The model under review builds one solid part; all positions refer to its coordinate system, in mm. A direction names the side the tool comes from. Round coordinates to 2 decimals unless told otherwise and drop trailing zeros. Write each loop counter-clockwise with the first axis right and the second up, starting at its lowest first coordinate (ties: lowest second). Pieces come first, ordered by that corner, then holes. Notation, with made-up numbers: (-1.75, 75.25) -> (38.25, 75.25) arc R19 ccw to (38.25, 110.25) -> close; hole circle Ø9 at (-9, 75). An arc over 180 degrees is marked (long way). Answer as a JSON object with one key per item and string values. Group by question number.
1) Insertion check: pin 1 Ø3 at (y, z) = (3, 18) entering from -X; pin 2 Ø3 at (x, y) = (4, 3) entering from +Z; pin 3 Ø3 at (x, y) = (5.5, 5) entering from +Z. Each pin has a flat end and moves straight along its axis. Give the tip position at first contact, or say it passes through.
2) Mouldability with a two-part tool opening along Z and no side actions: class faces 3 (the flat face through (-20, 6.35, -1)), 4 (the cylindrical face through (37.26, 3.13, -12.29)), 5 (the cylindrical face through (-46.492, 3.131, -10.324)) as pulls with the +Z half, pulls with the -Z half, needs draft (parallel to the pull), parting line crosses it, or undercut.
3) Machinability: for faces 1 (the cylindrical face through (12.495, 3.219, -22.057)), 2 (the flat face through (-20, 0, -1)), which of the approach directions +Z, -Z, +X, -X, +Y, -Y give a long, thin tool a straight path to every point of the face, cutting with its end or side? Answer none if there is none.
4) To check wall thickness, follow probe 1 along X at (y, z) = (2.5, 0) (3 decimals); probe 2 along X at (y, z) = (5.5, -12); probe 3 along Z at (x, y) = (6, 3.5). State the ranges of each line that lie inside material, in increasing order. Write a range as [from, to].
5) We need section D-D, the plane y = 3.5. Write out the cut boundary in (x, z) (3 decimals).
6) We need section B-B, the plane z = 0. Write out the cut boundary in (x, y) (3 decimals).
7) We need section C-C, the plane z = 15.5. Write out the cut boundary in (x, y).
8) We need section A-A, the plane x = 0. Write out the cut boundary in (y, z) (3 decimals).
from build123d import *

# Parameters (mm, degrees)
SKETCH2_R                = 47.625
SKETCH2_R_2              = 19
BOSS_EXTRUDE1_DEPTH      = 6.35
CUT_EXTRUDE1_DEPTH       = 68.650600515
FILLET1_R                = 6.35
CIRPATTERN1_COUNT        = 3
FILLET1_OF_CIRPATTERN1_R = 6.35


with BuildPart() as part:
    # Sketch2 → Boss-Extrude1 (new body)
    with BuildSketch(Plane(origin=(0, 0, 0), x_dir=(1, 0, 0), z_dir=(0, 1, 0))):
        with Locations(Location((0, 0, 0), (0, 0, 270))):
            Circle(SKETCH2_R)
        with Locations(Location((0, 0, 0), (0, 0, 270))):
            Circle(SKETCH2_R_2, mode=Mode.SUBTRACT)
    extrude(amount=BOSS_EXTRUDE1_DEPTH)

    # Sketch3 → Cut-Extrude1 (cut, through all)
    with BuildSketch(Plane(origin=(0, 6.35, 0), x_dir=(1, 0, 0), z_dir=(0, 1, 0))):
        with BuildLine():
            Line((24.486219696, 6.561062793), (39.86858848, 10.682756087))
            ThreePointArc((39.86858848, 10.682756087), (20.6375, 35.745198541), (-10.682756087, 39.86858848))
            Line((-10.682756087, 39.86858848), (-6.561062793, 24.486219696))
            ThreePointArc((-6.561062793, 24.486219696), (12.675, 21.953743986), (24.486219696, 6.561062793))
        make_face()
    cut_extrude1 = extrude(amount=-CUT_EXTRUDE1_DEPTH, mode=Mode.SUBTRACT)

    # Fillet1
    fillet1_edges = [part.edges().sort_by_distance(p)[0] for p in [
        (24.486219696, 3.175, -6.561062793),
        (-6.561062793, 3.175, -24.486219696),
        (-10.682756087, 3.175, -39.86858848),
        (39.86858848, 3.175, -10.682756087),
    ]]
    fillet(fillet1_edges, radius=FILLET1_R)

    # CirPattern1: Cut-Extrude1 ×3 about axis
    cirpattern1_axis = Axis((0, 0, 0), (0, 1, 0))
    for i in range(1, CIRPATTERN1_COUNT):
        add(cut_extrude1.rotate(cirpattern1_axis, i * 360 / CIRPATTERN1_COUNT), mode=Mode.SUBTRACT)

    # Fillet1 of CirPattern1
    fillet1_of_cirpattern1_edges = [part.edges().sort_by_distance(p)[0] for p in [
        (-17.925156903, 3.175, -17.925156903),
        (-17.925156903, 3.175, 17.925156903),
        (-29.185832393, 3.175, 29.185832393),
        (-29.185832393, 3.175, -29.185832393),
        (-6.561062793, 3.175, 24.486219696),
        (24.486219696, 3.175, 6.561062793),
        (39.86858848, 3.175, 10.682756087),
        (-10.682756087, 3.175, 39.86858848),
    ]]
    fillet(fillet1_of_cirpattern1_edges, radius=FILLET1_OF_CIRPATTERN1_R)


solid = part.part
Here are the results:
{
 "1": {"pin 1": "stops at x = -44.68", "pin 2": "stops at z = 47.56", "pin 3": "stops at z = 47.46"},
 "2": {"face 3": "needs draft", "face 4": "undercut", "face 5": "parting line crosses it"},
 "3": {"face 1": "+Y, -Y", "face 2": "+Z, -Z, +X, -X, -Y"},
 "4": {"probe 1": "x = [-47.625, -41.275], [-25.35, -19], [19, 47.625]", "probe 2": "x = [-46.09, -39.49], [-22.33, -14.73], [14.73, 22.33], [37.11, 46.09]", "probe 3": "z = [-47.25, -40.84], [-24.63, -18.03], [18.03, 24.63], [40.84, 47.25]"},
 "5": {"outline": "circle Ø95.25 at (0, 0); hole (-34.006, -23.393) arc R6.35 ccw to (-24.284, -24.284) -> (-21.961, -21.961) arc R6.35 ccw to (-21.153, -13.971) arc R25.35 cw to (-21.153, 13.971) arc R6.35 ccw to (-21.961, 21.961) -> (-24.284, 24.284) arc R6.35 ccw to (-34.006, 23.393) arc R41.275 ccw to start; hole circle Ø38 at (0, 0); hole (-8.889, -33.173) arc R6.35 ccw to (-3.256, -41.146) arc R41.275 ccw to (37.262, -17.754) arc R6.35 ccw to (33.173, -8.889) -> (29.999, -8.038) arc R6.35 ccw to (22.676, -11.333) arc R25.35 cw to (-1.523, -25.304) arc R6.35 ccw to (-8.038, -29.999) -> close; hole (-8.889, 33.173) -> (-8.038, 29.999) arc R6.35 ccw to (-1.523, 25.304) arc R25.35 cw to (22.676, 11.333) arc R6.35 ccw to (29.999, 8.038) -> (33.173, 8.889) arc R6.35 ccw to (37.262, 17.754) arc R41.275 ccw to (-3.256, 41.146) arc R6.35 ccw to start"},
 "6": {"outline": "(-47.625, 0) -> (-41.275, 0) -> (-41.275, 6.35) -> (-47.625, 6.35) -> close; (-25.35, 0) -> (-19, 0) -> (-19, 6.35) -> (-25.35, 6.35) -> close; (19, 0) -> (47.625, 0) -> (47.625, 6.35) -> (19, 6.35) -> close"},
 "7": {"outline": "(-45.03, 0) -> (-38.25, 0) -> (-38.25, 6.35) -> (-45.03, 6.35) -> close; (-20.41, 0) -> (-10.99, 0) -> (-10.99, 6.35) -> (-20.41, 6.35) -> close; (10.99, 0) -> (20.06, 0) -> (20.06, 6.35) -> (10.99, 6.35) -> close; (37.86, 0) -> (45.03, 0) -> (45.03, 6.35) -> (37.86, 6.35) -> close"},
 "8": {"outline": "(0, -47.625) -> (6.35, -47.625) -> (6.35, -41.275) -> (0, -41.275) -> close; (0, -25.35) -> (6.35, -25.35) -> (6.35, -19) -> (0, -19) -> close; (0, 19) -> (6.35, 19) -> (6.35, 25.35) -> (0, 25.35) -> close; (0, 41.275) -> (6.35, 41.275) -> (6.35, 47.625) -> (0, 47.625) -> close"}
}
